```python
from build123d import *

# Parameters (mm, degrees)
SKETCH_1_R      = 1.5
SKETCH_1_R_2    = 1.25
SKETCH_1_R_3    = 3.2
EXTRUDE_1_DEPTH = 2


with BuildPart() as part:
    # 草图1 → 凸台-拉伸1 (new body)
    with BuildSketch(Plane(origin=(0, 0, 0), x_dir=(1, 0, 0), z_dir=(0, 1, 0))):
        with BuildLine():
            Line((-20, 67.25), (-20, 51.25))
            Line((-20, 51.25), (-36, 51.25))
            ThreePointArc((-36, 51.25), (-38.828427125, 50.078427125), (-40, 47.25))
            Line((-40, 47.25), (-40, -47.25))
            ThreePointArc((-40, -47.25), (-38.828427125, -50.078427125), (-36, -51.25))
            Line((-36, -51.25), (36, -51.25))
            ThreePointArc((36, -51.25), (38.828427125, -50.078427125), (40, -47.25))
            Line((40, -47.25), (40, 47.25))
            ThreePointArc((40, 47.25), (38.828427125, 50.078427125), (36, 51.25))
            Line((36, 51.25), (20, 51.25))
            Line((20, 51.25), (20, 67.25))
            ThreePointArc((20, 67.25), (0, 87.25), (-20, 67.25))
        make_face()
        with Locations(Location((-28, 37, 0), (0, 0, 270))):
            Circle(SKETCH_1_R, mode=Mode.SUBTRACT)
        with Locations(Location((28, 37, 0), (0, 0, 270))):
            Circle(SKETCH_1_R, mode=Mode.SUBTRACT)
        with Locations(Location((-28, -37, 0), (0, 0, 270))):
            Circle(SKETCH_1_R, mode=Mode.SUBTRACT)
        with Locations(Location((28, -37, 0), (0, 0, 270))):
            Circle(SKETCH_1_R, mode=Mode.SUBTRACT)
        with Locations(Location((-20, 30, 0), (0, 0, 270))):
            Circle(SKETCH_1_R_2, mode=Mode.SUBTRACT)
        with Locations(Location((20, 30, 0), (0, 0, 270))):
            Circle(SKETCH_1_R_2, mode=Mode.SUBTRACT)
        with Locations(Location((-20, -30, 0), (0, 0, 270))):
            Circle(SKETCH_1_R_2, mode=Mode.SUBTRACT)
        with Locations(Location((20, -30, 0), (0, 0, 270))):
            Circle(SKETCH_1_R_2, mode=Mode.SUBTRACT)
        with Locations(Location((37, -37, 0), (0, 0, 270))):
            Circle(SKETCH_1_R, mode=Mode.SUBTRACT)
        with Locations(Location((-37, -37, 0), (0, 0, 270))):
            Circle(SKETCH_1_R, mode=Mode.SUBTRACT)
        with Locations(Location((-37, 37, 0), (0, 0, 270))):
            Circle(SKETCH_1_R, mode=Mode.SUBTRACT)
        with Locations(Location((37, 37, 0), (0, 0, 270))):
            Circle(SKETCH_1_R, mode=Mode.SUBTRACT)
        with Locations(Location((0, 67.25, 0), (0, 0, 270))):
            Circle(SKETCH_1_R_3, mode=Mode.SUBTRACT)
        with Locations(Location((0, 83.75, 0), (0, 0, 270))):
            Circle(SKETCH_1_R, mode=Mode.SUBTRACT)
        with Locations(Location((14.289419162, 59, 0), (0, 0, 270))):
            Circle(SKETCH_1_R, mode=Mode.SUBTRACT)
        with Locations(Location((-14.289419162, 59, 0), (0, 0, 270))):
            Circle(SKETCH_1_R, mode=Mode.SUBTRACT)
        with Locations(Location((-18, 24, 0), (0, 0, 270))):
            Circle(SKETCH_1_R, mode=Mode.SUBTRACT)
        with Locations(Location((18, 24, 0), (0, 0, 270))):
            Circle(SKETCH_1_R, mode=Mode.SUBTRACT)
        with Locations(Location((-18, -24, 0), (0, 0, 270))):
            Circle(SKETCH_1_R, mode=Mode.SUBTRACT)
        with Locations(Location((18, -24, 0), (0, 0, 270))):
            Circle(SKETCH_1_R, mode=Mode.SUBTRACT)
        with BuildLine():
            Line((-22.5, 47), (22.5, 47))
            ThreePointArc((22.5, 47), (24.5, 45), (22.5, 43))
            Line((22.5, 43), (-22.5, 43))
            ThreePointArc((-22.5, 43), (-24.5, 45), (-22.5, 47))
        make_face(mode=Mode.SUBTRACT)
        with BuildLine():
            Line((-13.531105432, 35), (13.531105432, 35))
            ThreePointArc((13.531105432, 35), (15.263754427, 33.998963192), (15.261958003, 31.997927459))
            Line((15.261958003, 31.997927459), (6.577747476, 16.997927459))
            ThreePointArc((6.577747476, 16.997927459), (5.845858097, 16.267351005), (4.846894905, 16))
            Line((4.846894905, 16), (-4.846894905, 16))
            ThreePointArc((-4.846894905, 16), (-5.845858097, 16.267351005), (-6.577747476, 16.997927459))
            Line((-6.577747476, 16.997927459), (-15.261958003, 31.997927459))
            ThreePointArc((-15.261958003, 31.997927459), (-15.263754427, 33.998963192), (-13.531105432, 35))
        make_face(mode=Mode.SUBTRACT)
        with BuildLine():
            Line((16.585786438, 11.585786438), (28.585786438, 23.585786438))
            ThreePointArc((28.585786438, 23.585786438), (30.765366865, 24.01933194), (32, 22.171572875))
            Line((32, 22.171572875), (32, -22.171572875))
            ThreePointArc((32, -22.171572875), (30.765366865, -24.01933194), (28.585786438, -23.585786438))
            Line((28.585786438, -23.585786438), (16.585786438, -11.585786438))
            ThreePointArc((16.585786438, -11.585786438), (16.152240935, -10.93693974), (16, -10.171572875))
            Line((16, -10.171572875), (16, 10.171572875))
            ThreePointArc((16, 10.171572875), (16.152240935, 10.93693974), (16.585786438, 11.585786438))
        make_face(mode=Mode.SUBTRACT)
        with BuildLine():
            Line((4.846894905, -16), (-4.846894905, -16))
            ThreePointArc((-4.846894905, -16), (-5.845858097, -16.267351005), (-6.577747476, -16.997927459))
            Line((-6.577747476, -16.997927459), (-15.261958003, -31.997927459))
            ThreePointArc((-15.261958003, -31.997927459), (-15.263754427, -33.998963192), (-13.531105432, -35))
            Line((-13.531105432, -35), (13.531105432, -35))
            ThreePointArc((13.531105432, -35), (15.263754427, -33.998963192), (15.261958003, -31.997927459))
            Line((15.261958003, -31.997927459), (6.577747476, -16.997927459))
            ThreePointArc((6.577747476, -16.997927459), (5.845858097, -16.267351005), (4.846894905, -16))
        make_face(mode=Mode.SUBTRACT)
        with BuildLine():
            Line((-16.585786438, -11.585786438), (-28.585786438, -23.585786438))
            ThreePointArc((-28.585786438, -23.585786438), (-30.765366865, -24.01933194), (-32, -22.171572875))
            Line((-32, -22.171572875), (-32, 22.171572875))
            ThreePointArc((-32, 22.171572875), (-30.765366865, 24.01933194), (-28.585786438, 23.585786438))
            Line((-28.585786438, 23.585786438), (-16.585786438, 11.585786438))
            ThreePointArc((-16.585786438, 11.585786438), (-16.152240935, 10.93693974), (-16, 10.171572875))
            Line((-16, 10.171572875), (-16, -10.171572875))
            ThreePointArc((-16, -10.171572875), (-16.152240935, -10.93693974), (-16.585786438, -11.585786438))
        make_face(mode=Mode.SUBTRACT)
        with BuildLine():
            Line((-6, -9), (6, -9))
            ThreePointArc((6, -9), (8.121320344, -8.121320344), (9, -6))
            Line((9, -6), (9, 6))
            ThreePointArc((9, 6), (8.121320344, 8.121320344), (6, 9))
            Line((6, 9), (-6, 9))
            ThreePointArc((-6, 9), (-8.121320344, 8.121320344), (-9, 6))
            Line((-9, 6), (-9, -6))
            ThreePointArc((-9, -6), (-8.121320344, -8.121320344), (-6, -9))
        make_face(mode=Mode.SUBTRACT)
        with BuildLine():
            Line((-22.5, -43), (22.5, -43))
            ThreePointArc((22.5, -43), (24.5, -45), (22.5, -47))
            Line((22.5, -47), (-22.5, -47))
            ThreePointArc((-22.5, -47), (-24.5, -45), (-22.5, -43))
        make_face(mode=Mode.SUBTRACT)
        with BuildLine():
            ThreePointArc((4.5, 75.044228634), (7.794228634, 71.75), (9, 67.25))
            ThreePointArc((9, 67.25), (10.5, 65.75), (12, 67.25))
            ThreePointArc((12, 67.25), (10.392304845, 73.25), (6, 77.642304845))
            ThreePointArc((6, 77.642304845), (3.950961894, 77.09326674), (4.5, 75.044228634))
        make_face(mode=Mode.SUBTRACT)
        with BuildLine():
            ThreePointArc((-6, 56.857695155), (-6.549038106, 58.90673326), (-4.5, 59.455771366))
            ThreePointArc((-4.5, 59.455771366), (0, 58.25), (4.5, 59.455771366))
            ThreePointArc((4.5, 59.455771366), (6.549038106, 58.90673326), (6, 56.857695155))
            ThreePointArc((6, 56.857695155), (0, 55.25), (-6, 56.857695155))
        make_face(mode=Mode.SUBTRACT)
        with BuildLine():
            ThreePointArc((-6, 77.642304845), (-3.950961894, 77.09326674), (-4.5, 75.044228634))
            ThreePointArc((-4.5, 75.044228634), (-7.794228634, 71.75), (-9, 67.25))
            ThreePointArc((-9, 67.25), (-10.5, 65.75), (-12, 67.25))
            ThreePointArc((-12, 67.25), (-10.392304845, 73.25), (-6, 77.642304845))
        make_face(mode=Mode.SUBTRACT)
    extrude(amount=EXTRUDE_1_DEPTH)


solid = part.part
```
Design review of the part built by this model. Coordinates are the model's own, in mm. A direction names the side the tool comes from. Coordinates: 2 decimals unless noted, no trailing zeros. Write each loop counter-clockwise with the first axis right and the second up, starting at its lowest first coordinate (ties: lowest second). Pieces come first, ordered by that corner, then holes. Notation, with made-up numbers: M 37,-31 L 53,-31 A17 ccw 53,2 Z; hole C 58,88.25 d7. An arc over 180 degrees is marked long. Answer as a JSON object with one key per item and string values.
Item 1: Wall thickness on probe 1 along X at (y, z) = (1.8, 10); probe 2 along X at (y, z) = (0.7, -37); probe 3 along X at (y, z) = (0.8, 2): over which ranges is each line inside the solid? List them lowest first.
Outcome:
{"probe 1": "-40 to -32, -16 to 16, 32 to 40", "probe 2": "-40 to -38.5, -35.5 to -29.5, -26.5 to 26.5, 29.5 to 35.5, 38.5 to 40", "probe 3": "-40 to -32, -16 to -9, 9 to 16, 32 to 40"}
Item 2: Add section C-C, the plane z = -83.75. Give the boundary of the cut face in (x, y).
Outcome:
{"outline": "M -11.3,0 L -1.5,0 L -1.5,2 L -11.3,2 Z; M 1.5,0 L 11.3,0 L 11.3,2 L 1.5,2 Z"}
Item 3: Insertion check: pin 1 Ø1.8 at (x, z) = (-37, 37) entering from +Y; pin 2 Ø0.6 at (x, y) = (-2.5, 1) entering from -Z; pin 3 Ø1 at (x, y) = (-27.5, 0.5) entering from -Z. Each pin has a flat end and moves straight along its axis. Give the tip position at first contact, or say it passes through.
Outcome:
{"pin 1": "through", "pin 2": "z = -87.13", "pin 3": "z = -51.25"}
Item 4: Add section D-D, the plane z = -69. Give the boundary of the cut face in (x, y).
Outcome:
{"outline": "M -19.92,0 L -11.87,0 L -11.87,2 L -19.92,2 Z; M -8.83,0 L -2.68,0 L -2.68,2 L -8.83,2 Z; M 2.68,0 L 8.83,0 L 8.83,2 L 2.68,2 Z; M 11.87,0 L 19.92,0 L 19.92,2 L 11.87,2 Z"}
Item 5: Add section A-A, the plane z = 14. Give the boundary of the cut face in (x, y), and give its area (3 significant figures).
Outcome:
{"outline": "M -40,0 L -32,0 L -32,2 L -40,2 Z; M -19,0 L 19,0 L 19,2 L -19,2 Z; M 32,0 L 40,0 L 40,2 L 32,2 Z", "area": "108 mm²"}
Item 6: Draft analysis for pull direction X (two halves, no side actions). For faces 3 (the cylindrical face through (-37.9, 1, -38.2)), 4 (the cylindrical face through (-10.44, 0.99, -73.17)), 5 (the flat face through (-9, 0, -19)), 6 (the cylindrical face through (-38.859, 0.986, 50.047)), state which applies: pulls with the +X half, pulls with the -X half, needs draft (parallel to the pull), parting line crosses it, or undercut.
Outcome:
{"face 3": "undercut", "face 4": "undercut", "face 5": "needs draft", "face 6": "pulls with the -X half"}
Item 7: Add section B-B, the plane z = 37. Give the boundary of the cut face in (x, y).
Outcome:
{"outline": "M -40,0 L -38.5,0 L -38.5,2 L -40,2 Z; M -35.5,0 L -29.5,0 L -29.5,2 L -35.5,2 Z; M -26.5,0 L 26.5,0 L 26.5,2 L -26.5,2 Z; M 29.5,0 L 35.5,0 L 35.5,2 L 29.5,2 Z; M 38.5,0 L 40,0 L 40,2 L 38.5,2 Z"}
Item 8: Machinability: for faces 1 (the flat face through (23, 1, 18)), 2 (the flat face through (-9, 2, -19)), which of the approach directions +Z, -Z, +X, -X, +Y, -Y give a long, thin tool a straight path to every point of the face, cutting with its end or side? Answer none if there is none.
Outcome:
{"face 1": "+Y, -Y", "face 2": "+Z, -Z, +X, -X, +Y"}
